```python
from build123d import *

# Parameters (mm, degrees)
BOSS_EXTRUDE1_DEPTH = 5
SKETCH2_W           = 2.5
SKETCH2_H           = 2.5
BOSS_EXTRUDE2_DEPTH = 5
SKETCH3_W           = 3
SKETCH3_H           = 3
CUT_EXTRUDE1_DEPTH  = 21


with BuildPart() as part:
    # Sketch1 → Boss-Extrude1 (new body)
    with BuildSketch(Plane.XY):
        Polygon((0, 6.7), (0, 8.05), (5.5, 8.05), (14.2, 8.05), (14.2, -18.95), (146.5, -18.95), (146.5, -13.95), (19.2, -13.95), (19.2, 12.9), (5.5, 12.9), (-5, 12.9), (-5, 0), (0, 0), align=None)
    extrude(amount=BOSS_EXTRUDE1_DEPTH)

    # Sketch2 → Boss-Extrude2 (add)
    with BuildSketch(Plane(origin=(146.5, 0, 0), x_dir=(0, 0, -1), z_dir=(1, 0, 0))):
        with Locations((-2.5, -16.45)):
            Rectangle(SKETCH2_W, SKETCH2_H)
    extrude(amount=BOSS_EXTRUDE2_DEPTH)

    # Sketch3 → Cut-Extrude1 (cut)
    with BuildSketch(Plane.XY.offset(5)):
        with Locations((80.35, -16.45)):
            Rectangle(SKETCH3_W, SKETCH3_H)
    extrude(amount=-CUT_EXTRUDE1_DEPTH, mode=Mode.SUBTRACT)


solid = part.part
```
Read the model definition and answer for the solid it produces. Units are mm, in the model's axes. A direction names the side the tool comes from. Coordinates: 2 decimals unless noted, no trailing zeros. Loops run counter-clockwise (first coordinate to the right, second up) from the corner with the lowest first, then second, coordinate; pieces in that order, holes last. Notation, with made-up numbers: (28, 5) - (86, 5) arc R30 cw to (86, 37) - close; hole circle Ø9 at (30, -29). An arc over 180 degrees is marked (long way). Answer in a Markdown table with one row per item.
1. Which of the six approach directions +Z, -Z, +X, -X, +Y, -Y give full straight-line access (tool end or side, diameter ignored) to faces 4 (the face through (19.2, -1, 2)), 5 (the face through (149, -16, 1.25)), 6 (the face through (149, -16, 3.75)), 7 (the face through (80, -14.95, 3)), 8 (the face through (14.2, -5, 2))?
Conclusion:
| item | result |
|---|---|
| face 4 | +Z, -Z, +X, +Y |
| face 5 | -Z, +X, +Y, -Y |
| face 6 | +Z, +X, +Y, -Y |
| face 7 | +Z, -Z |
| face 8 | +Z, -Z, -Y |
2. Find section D-D, the plane x = 131. Write down the section's boundary in (y, z).
Conclusion:
| item | result |
|---|---|
| outline | (-18.95, 0) - (-13.95, 0) - (-13.95, 5) - (-18.95, 5) - close |
3. Find section C-C, the plane y = -6. Write down the section's boundary in (x, z).
Conclusion:
| item | result |
|---|---|
| outline | (14.2, 0) - (19.2, 0) - (19.2, 5) - (14.2, 5) - close |
4. Determine the mould class of faces 1 (the face through (79, -18.95, 2)), 2 (the face through (80, -17.95, 3)), 3 (the face through (-5, 7, 2)) for opening direction X: +X half, -X half, draft (parallel to the pull), parting line (faces both ways), or undercut.
Conclusion:
| item | result |
|---|---|
| face 1 | draft |
| face 2 | undercut |
| face 3 | -X half |
5. Straight lines are drawn through the part: line 1 (X direction, y = -15, z = 1.5); line 2 (X direction, y = 7.5, z = 1); line 3 (Y direction, x = 83.5, z = 2.7). For each, find the intervals that lie inside material, in ascending order.
Conclusion:
| item | result |
|---|---|
| line 1 | x = 14.2 to 78.85, 81.85 to 146.5 |
| line 2 | x = -5 to 0, 14.2 to 19.2 |
| line 3 | y = -18.95 to -13.95 |
6. Given pin 1 (1.2 mm diameter, centred on x = 148.5, y = -16, fed in from +Z); pin 2 (2 mm diameter, centred on x = 148.5, z = 2, fed in from +Y); pin 3 (2.5 mm diameter, centred on x = 10, z = 2, fed in from -Y); pin 4 (6 mm diameter, centred on x = 12.5, y = 7, fed in from +Z), each flat-ended and moving along its own axis, determine where each tip first touches the part or whether it passes through.
Conclusion:
| item | result |
|---|---|
| pin 1 | stops at z = 3.75 |
| pin 2 | stops at y = -15.2 |
| pin 3 | stops at y = 8.05 |
| pin 4 | stops at z = 5 |
7. Find section A-A, the plane y = 5. Write down the section's boundary in (x, z).
Conclusion:
| item | result |
|---|---|
| outline | (-5, 0) - (0, 0) - (0, 5) - (-5, 5) - close; (14.2, 0) - (19.2, 0) - (19.2, 5) - (14.2, 5) - close |
8. Find section B-B, the plane z = 2.3. Write down the section's boundary in (x, y).
Conclusion:
| item | result |
|---|---|
| outline | (-5, 0) - (0, 0) - (0, 8.05) - (14.2, 8.05) - (14.2, -18.95) - (146.5, -18.95) - (146.5, -17.7) - (151.5, -17.7) - (151.5, -15.2) - (146.5, -15.2) - (146.5, -13.95) - (19.2, -13.95) - (19.2, 12.9) - (-5, 12.9) - close; hole (78.85, -17.95) - (81.85, -17.95) - (81.85, -14.95) - (78.85, -14.95) - close |
